Verification items for the finished model (mm, model axes). Face numbers are marked on the shaded views. A direction names the side the tool comes from. Coordinates: 2 decimals unless noted, no trailing zeros. Write each loop counter-clockwise with the first axis right and the second up, starting at its lowest first coordinate (ties: lowest second). Pieces come first, ordered by that corner, then holes.
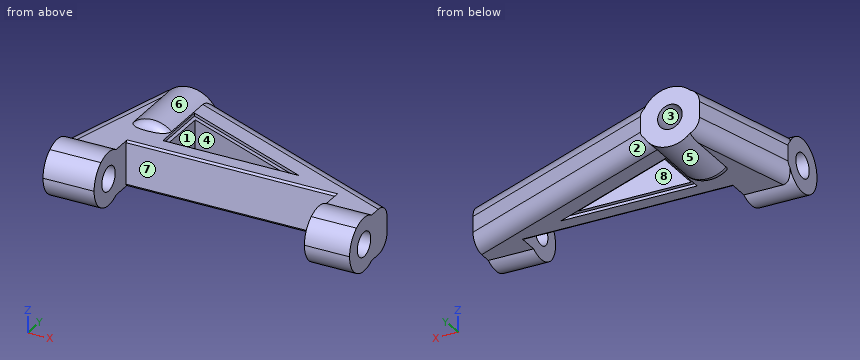
```python
from build123d import *

# Parameters (mm, degrees)
EXTRUDE_1_DEPTH        = 4.6
SKETCH_2_R             = 3
EXTRUDE_2_DEPTH        = 8
SKETCH_3_R             = 2.7
EXTRUDE_3_DEPTH        = 5.2
SKETCH_5_R             = 2.7
EXTRUDE_4_DEPTH        = 4.6
CUT_EXTRUDE_1_DEPTH    = 35.524918537
FILLET_1_R             = 1.5
CUT_EXTRUDE_2_DEPTH    = 30.215920451
CUT_EXTRUDE_3_DEPTH    = 0.3
CUT_EXTRUDE_4_DEPTH    = 0.3
FILLET_2_R             = 0.2
FILLET_3_R             = 1
SKETCH_9_R             = 1.25
CUT_EXTRUDE_5_DEPTH    = 35.524918683
HOLE_WIZARD_M3_1_D     = 2.5
HOLE_WIZARD_M3_1_DEPTH = 6.5
HOLE_WIZARD_M3_1_TIP   = 0.751075774


with BuildPart() as part:
    # 草图1 → 凸台-拉伸1 (new body)
    with BuildSketch(Plane.XY):
        Polygon((-0.8, -2.7), (-0.8, 3.3), (20.6, 3.3), (20.6, -2.7), (25.2, -2.7), (25.2, 4.3), (3, 13.8), (-3, 13.8), (-6, 2.7), (-6, -2.7), align=None)
        Polygon((2.46680021, 10.221171171), (2.46680021, 5.3), (13.96680021, 5.3), align=None, mode=Mode.SUBTRACT)
    extrude(amount=EXTRUDE_1_DEPTH)

    # 草图2 → 凸台-拉伸2 (add)
    with BuildSketch(Plane(origin=(0, 13.8, 0), x_dir=(1, 0, 0), z_dir=(0, 1, 0))):
        with Locations((0, -2.3)):
            Circle(SKETCH_2_R)
    extrude(amount=-EXTRUDE_2_DEPTH)

    # 草图3 → 凸台-拉伸3 (add)
    with BuildSketch(Plane.ZY.offset(6)):
        with Locations((2.3, 0)):
            Circle(SKETCH_3_R)
    extrude(amount=-EXTRUDE_3_DEPTH)

    # 草图5 → 凸台-拉伸4 (add)
    with BuildSketch(Plane.ZY.offset(-20.6)):
        with Locations((2.3, 0)):
            Circle(SKETCH_5_R)
    extrude(amount=-EXTRUDE_4_DEPTH)

    # 草图4 → 切除-拉伸1 (cut, through all)
    with BuildSketch(Plane.ZY.offset(6)):
        with BuildLine():
            ThreePointArc((4.6, -1.414213562), (3.617502065, -2.356732549), (2.3, -2.7))
            Line((2.3, -2.7), (4.6, -2.7))
            Line((4.6, -2.7), (4.6, -1.414213562))
        make_face()
        with BuildLine():
            ThreePointArc((2.3, -2.7), (0.982497935, -2.356732549), (0, -1.414213562))
            Line((0, -1.414213562), (0, -2.7))
            Line((0, -2.7), (2.3, -2.7))
        make_face()
    extrude(amount=-CUT_EXTRUDE_1_DEPTH, mode=Mode.SUBTRACT)

    # 圆角1
    # the kernel refuses this fillet: 1.5 mm, written as the material it takes off along each edge
    with BuildSketch(Plane(origin=(-2.021591156, 17.420112724, 0), x_dir=(0.9653633930282662, -0.26090902514277475, 0), z_dir=(-0.2609090251427748, -0.9653633930282663, 0))) as fillet_1_piece_1_section:
        with BuildLine():
            CenterArc((FILLET_1_R, FILLET_1_R), FILLET_1_R, 180, 90)
            Line((0, FILLET_1_R), (0, 0))
            Line((0, 0), (FILLET_1_R, 0))
        make_face()
    fillet_1_piece_1 = extrude(amount=18.998260738, mode=Mode.PRIVATE)
    fillet_1_piece_1 = fillet_1_piece_1 - Plane(origin=(-4.247071053, 0, 2.3), x_dir=(0, 0, 1), z_dir=(-1, 0, 0)) * Cylinder(2.7, 44, mode=Mode.PRIVATE)
    fillet_1_piece_1 = fillet_1_piece_1 - Plane(origin=(0, 7.876054914, 2.3), x_dir=(1, 0, 0), z_dir=(0, 1, 0)) * Cylinder(3, 44, mode=Mode.PRIVATE)
    add(fillet_1_piece_1, mode=Mode.SUBTRACT)
    with BuildSketch(Plane(origin=(-2.021591156, 17.420112724, 4.6), x_dir=(0.9653633930282662, -0.26090902514277475, 0), z_dir=(-0.2609090251427748, -0.9653633930282663, 0))) as fillet_1_piece_2_section:
        with BuildLine():
            CenterArc((FILLET_1_R, -FILLET_1_R), FILLET_1_R, 90, 90)
            Line((0, -FILLET_1_R), (0, 0))
            Line((0, 0), (FILLET_1_R, 0))
        make_face()
    fillet_1_piece_2 = extrude(amount=18.998260738, mode=Mode.PRIVATE)
    fillet_1_piece_2 = fillet_1_piece_2 - Plane(origin=(-4.247069139, 0, 2.3), x_dir=(0, 0, 1), z_dir=(-1, 0, 0)) * Cylinder(2.7, 44, mode=Mode.PRIVATE)
    fillet_1_piece_2 = fillet_1_piece_2 - Plane(origin=(0, 7.876066276, 2.3), x_dir=(1, 0, 0), z_dir=(0, 1, 0)) * Cylinder(3, 44, mode=Mode.PRIVATE)
    add(fillet_1_piece_2, mode=Mode.SUBTRACT)
    with BuildSketch(Plane(origin=(28.647596614, 2.824677125, 0), x_dir=(-0.39341943343746105, -0.9193590970854355, 0), z_dir=(-0.9193590970854355, 0.39341943343746105, 0))) as fillet_1_piece_3_section:
        with BuildLine():
            CenterArc((FILLET_1_R, FILLET_1_R), FILLET_1_R, 180, 90)
            Line((0, FILLET_1_R), (0, 0))
            Line((0, 0), (FILLET_1_R, 0))
        make_face()
    fillet_1_piece_3 = extrude(amount=31.647256573, mode=Mode.PRIVATE)
    fillet_1_piece_3 = fillet_1_piece_3 - Plane(origin=(0, 8.805883363, 2.3), x_dir=(1, 0, 0), z_dir=(0, 1, 0)) * Cylinder(3, 70, mode=Mode.PRIVATE)
    add(fillet_1_piece_3, mode=Mode.SUBTRACT)
    with BuildSketch(Plane(origin=(28.647596614, 2.824677125, 4.6), x_dir=(-0.39341943343746105, -0.9193590970854355, 0), z_dir=(-0.9193590970854355, 0.39341943343746105, 0))) as fillet_1_piece_4_section:
        with BuildLine():
            CenterArc((FILLET_1_R, -FILLET_1_R), FILLET_1_R, 90, 90)
            Line((0, -FILLET_1_R), (0, 0))
            Line((0, 0), (FILLET_1_R, 0))
        make_face()
    fillet_1_piece_4 = extrude(amount=31.647256573, mode=Mode.PRIVATE)
    fillet_1_piece_4 = fillet_1_piece_4 - Plane(origin=(0, 8.805887847, 2.3), x_dir=(1, 0, 0), z_dir=(0, 1, 0)) * Cylinder(3, 70, mode=Mode.PRIVATE)
    add(fillet_1_piece_4, mode=Mode.SUBTRACT)

    # 草图6 → 切除-拉伸2 (cut, through all)
    with BuildSketch(Plane.XY.offset(4.6)):
        Polygon((13.96680021, 5.3), (2.46680021, 10.221171171), (2.46680021, 5.3), align=None)
    extrude(amount=-CUT_EXTRUDE_2_DEPTH, mode=Mode.SUBTRACT)

    # 草图7 → 切除-拉伸3 (cut)
    with BuildSketch(Plane.XY.offset(4.6)):
        Polygon((2.06680021, 10.827428046), (2.06680021, 4.9), (15.918263645, 4.9), align=None)
        Polygon((2.46680021, 10.221171171), (2.46680021, 5.3), (13.96680021, 5.3), align=None, mode=Mode.SUBTRACT)
    extrude(amount=-CUT_EXTRUDE_3_DEPTH, mode=Mode.SUBTRACT)

    # 草图8 → 切除-拉伸4 (cut)
    with BuildSketch(Plane(origin=(0, 0, 0), x_dir=(-1, 0, 0), z_dir=(0, 0, -1))):
        Polygon((-2.06680021, 4.9), (-2.06680021, 10.827428046), (-15.918263645, 4.9), align=None)
        Polygon((-2.46680021, 5.3), (-2.46680021, 10.221171171), (-13.96680021, 5.3), align=None, mode=Mode.SUBTRACT)
    extrude(amount=-CUT_EXTRUDE_4_DEPTH, mode=Mode.SUBTRACT)

    # 圆角2
    fillet_2_edges = [part.edges().sort_by_distance(p)[0] for p in [
        (9.9, 3.3, 4.6),
        (9.9, 3.3, 0),
    ]]
    fillet(fillet_2_edges, radius=FILLET_2_R)

    # 圆角3
    # the kernel refuses this fillet: 1 mm, written as the material it takes off along each edge
    with BuildSketch(Plane(origin=(0, 5.8, 2.3), x_dir=(-0.9991986620043835, 0, 0.040025415034074786), z_dir=(-0.040025415034074786, 0, -0.9991986620043835))) as fillet_3_piece_1_section:
        with BuildLine():
            CenterArc((3 - FILLET_3_R, FILLET_3_R), FILLET_3_R, 270, 90)
            Line((3 - FILLET_3_R, 0), (3, 0))
            Line((3, 0), (3, FILLET_3_R))
        make_face()
    fillet_3_piece_1 = revolve(axis=Axis((0, 5.8, 2.3), (0, 1, 0)), revolution_arc=175.412199766, mode=Mode.PRIVATE)
    fillet_3_piece_1 = split(fillet_3_piece_1, bisect_by=Plane(origin=(0, 6.202737669, 4.6), z_dir=(0, 0, 1)), keep=Keep.TOP, mode=Mode.PRIVATE)
    add(fillet_3_piece_1, mode=Mode.SUBTRACT)
    with BuildSketch(Plane(origin=(0, 5.8, 2.3), x_dir=(0.9991986620043835, 0, -0.04002541503407598), z_dir=(0.04002541503407598, 0, 0.9991986620043835))) as fillet_3_piece_2_section:
        with BuildLine():
            CenterArc((3 - FILLET_3_R, FILLET_3_R), FILLET_3_R, 270, 90)
            Line((3 - FILLET_3_R, 0), (3, 0))
            Line((3, 0), (3, FILLET_3_R))
        make_face()
    fillet_3_piece_2 = revolve(axis=Axis((0, 5.8, 2.3), (0, 1, 0)), revolution_arc=175.412199766, mode=Mode.PRIVATE)
    fillet_3_piece_2 = split(fillet_3_piece_2, bisect_by=Plane(origin=(0, 6.202737669, 0), z_dir=(0, 0, -1)), keep=Keep.TOP, mode=Mode.PRIVATE)
    add(fillet_3_piece_2, mode=Mode.SUBTRACT)

    # 草图9 → 切除-拉伸5 (cut, through all)
    with BuildSketch(Plane.ZY.offset(6)):
        with Locations((2.3, 0)):
            Circle(SKETCH_9_R)
    extrude(amount=-CUT_EXTRUDE_5_DEPTH, mode=Mode.SUBTRACT)

    # M3 螺纹孔1
    with Locations(Plane(origin=(0, 13.8, 2.3), x_dir=(0, 0, 1), z_dir=(0, 1, 0))):
        with Locations((0, 0)):
            Hole(HOLE_WIZARD_M3_1_D / 2, depth=HOLE_WIZARD_M3_1_DEPTH)
            with Locations((0, 0, -(HOLE_WIZARD_M3_1_DEPTH + HOLE_WIZARD_M3_1_TIP / 2))):  # 118° drill point
                Cone(0, HOLE_WIZARD_M3_1_D / 2, HOLE_WIZARD_M3_1_TIP, mode=Mode.SUBTRACT)


solid = part.part
```
1. Tool access check on the marked faces 5, 6, 7 and 8. Record the directions out of +Z, -Z, +X, -X, +Y, -Y that give a thin tool (end or side, any length) a straight path to the whole face; none if there is none.
2. Material ranges on L1, parallel to Y at x = -2.8, z = 2.3; L2, parallel to X at y = 2, z = 1; L3, parallel to Z at x = 0, y = 9, recorded low to high.
3. Sectioned sample at A-A, the plane y = 0. Record the boundary of the cut face in (x, z), and give its area (3 significant figures).
4. Draft check along Y on the marked faces 1, 2, 3 and 4. Enter one of: pulls with the +Y half, pulls with the -Y half, needs draft (parallel to the pull), parting line crosses it, or undercut.
5. Sectioned sample at B-B, the plane y = 9. Give the number of separate pieces and of enclosed holes in the cut face, and give its area (3 significant figures).
6. Gauge pin test, flat ends, axial feed: P1, Ø1, axis at x = 5.5, z = 4.5, coming from the -Y side; P2, Ø3, axis at x = 7, z = 2, coming from the +Y side; P3, Ø5, axis at x = 11, y = 2.5, coming from the -Z side. Record the tip position at first contact, or that the pin passes through.
Outcome:
1. face 5: -Z, +Y
1. face 6: +Z, +Y
1. face 7: +Z, -Z, -Y
1. face 8: +Z, -Z
2. L1: y = -2.7 to -1.25, 1.25 to 13.8
2. L2: x = -6 to -0.8, 20.6 to 25.2
2. L3: z = -0.7 to 1.05, 3.55 to 5.3
3. outline: (-6, -0.4) - (-0.8, -0.4) - (-0.8, 1.05) - (-6, 1.05) - close; (-6, 3.55) - (-0.8, 3.55) - (-0.8, 5) - (-6, 5) - close; (20.6, -0.4) - (25.2, -0.4) - (25.2, 1.05) - (20.6, 1.05) - close; (20.6, 3.55) - (25.2, 3.55) - (25.2, 5) - (20.6, 5) - close
3. area: 28.4 mm2
4. face 1: undercut
4. face 2: pulls with the +Y half
4. face 3: needs draft
4. face 4: undercut
5. separate pieces: 2
5. enclosed holes: 1
5. area: 66.5 mm2
6. P1: stops at y = 3.3
6. P2: stops at y = 12.73
6. P3: stops at z = 0
